Check sheet for the drawn part. Datum: minimum x, y, z corner. Units: mm. Round coordinates to 2 decimals unless told otherwise and drop trailing zeros. Order: outer loops, then holes, each group sorted by start corner. A loop starts at its lowest first (then second) coordinate and runs counter-clockwise, first axis right, second up. Notation, with made-up numbers: (62, 81) -> (87, 81) arc R20 ccw to (87, 101) -> close; hole circle Ø2 at (85, 13). An arc over 180 degrees is marked (long way). Answer in a Markdown table with one row per item.
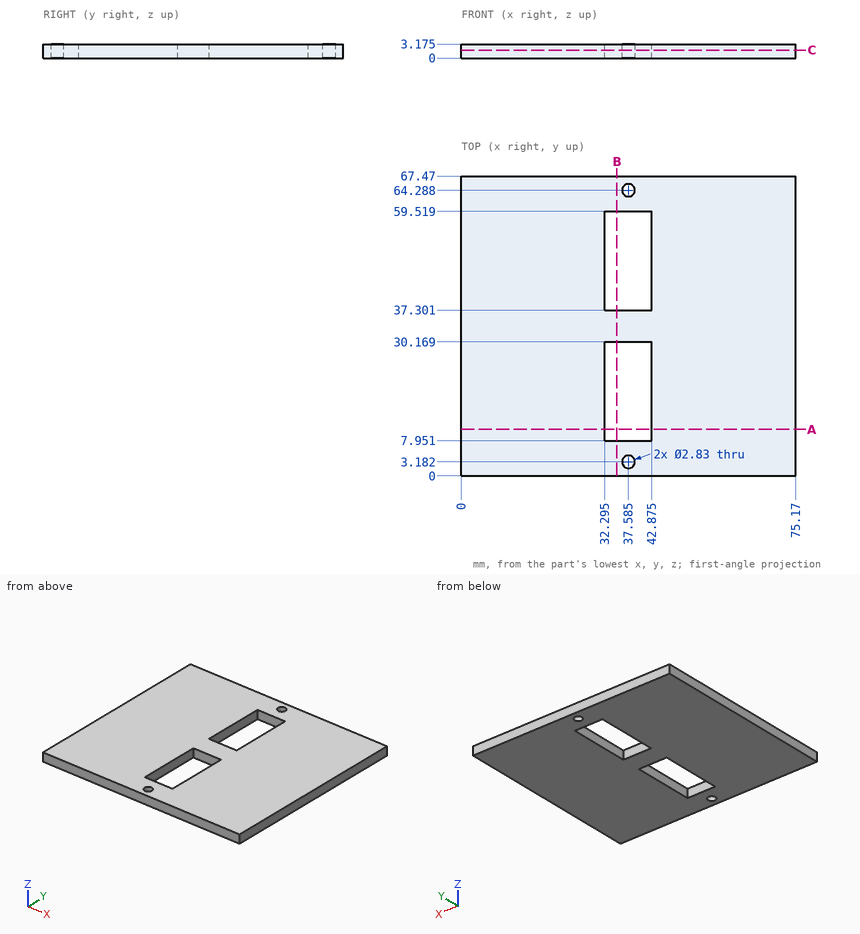
(1) Section check A-A on y = 10.5. Record the boundary of the cut face in (x, z) (3 decimals), plus the area to 3 significant figures.
Solutions:
| item | result |
|---|---|
| outline | (0, 0) -> (32.295, 0) -> (32.295, 3.175) -> (0, 3.175) -> close; (42.875, 0) -> (75.17, 0) -> (75.17, 3.175) -> (42.875, 3.175) -> close |
| area | 205 mm^2 |
(2) Section check C-C on z = 1.8. Record the boundary of the cut face in (x, y) (3 decimals), plus the area to 3 significant figures.
Solutions:
| item | result |
|---|---|
| outline | (0, 0) -> (75.17, 0) -> (75.17, 67.47) -> (0, 67.47) -> close; hole (32.295, 7.951) -> (42.875, 7.951) -> (42.875, 30.169) -> (32.295, 30.169) -> close; hole (32.295, 37.301) -> (42.875, 37.301) -> (42.875, 59.519) -> (32.295, 59.519) -> close; hole circle Ø2.83 at (37.585, 3.182); hole circle Ø2.83 at (37.585, 64.288) |
| area | 4,590 mm^2 |
(3) Scan lines: probe 1 along X at (y, z) = (59, 1.55) (3 decimals); probe 2 along X at (y, z) = (64.5, 2.8). Record each from-to range of solid material in increasing order. Write a range as from..to.
Solutions:
| item | result |
|---|---|
| probe 1 | 0..32.295, 42.875..75.17 |
| probe 2 | 0..36.19, 38.98..75.17 |
(4) Section check B-B on x = 35. Record the boundary of the cut face in (y, z) (3 decimals).
Solutions:
| item | result |
|---|---|
| outline | (0, 0) -> (7.951, 0) -> (7.951, 3.175) -> (0, 3.175) -> close; (30.169, 0) -> (37.301, 0) -> (37.301, 3.175) -> (30.169, 3.175) -> close; (59.519, 0) -> (67.47, 0) -> (67.47, 3.175) -> (59.519, 3.175) -> close |
